```python
from build123d import *

# Parameters (mm, degrees)
F0_W     = 50.8
F0_H     = 25.4
F0_W_2   = 44.45
F0_H_2   = 19.05
F1_DEPTH = 447.675
F2_R     = 3.2385
F2_R_2   = 2.579688
F2_R_3   = 3.175
F3_DEPTH = 25.4
F4_R     = 2.5781
F5_DEPTH = 50.801
F6_DEPTH = 76.2
F7_DEPTH = 25.4


with BuildPart() as f1:
    # F0 (on Front) → F1 (new body)
    with BuildSketch(Plane.XZ):
        with Locations((-27.201447, 17.172885)):
            Rectangle(F0_W, F0_H)
        with Locations((-27.201447, 17.172885)):
            Rectangle(F0_W_2, F0_H_2, mode=Mode.SUBTRACT)
    extrude(amount=F1_DEPTH)

    # F2 (on face) → F3 (cut)
    with BuildSketch(Plane.XY.offset(29.872885)):
        with Locations((-27.201447, -304.8)):
            Circle(F2_R)
        with Locations((-27.201447, -266.7)):
            Circle(F2_R)
        with Locations((-27.201447, -101.6)):
            Circle(F2_R)
        with Locations((-27.201447, -38.1)):
            Circle(F2_R)
        with Locations((-46.251447, -127)):
            Circle(F2_R_2)
        with Locations((-39.901447, -127)):
            Circle(F2_R_2)
        with Locations((-14.501447, -127)):
            Circle(F2_R_2)
        with Locations((-8.151447, -127)):
            Circle(F2_R_2)
        with Locations((-46.251447, -69.85)):
            Circle(F2_R_2)
        with Locations((-39.901447, -69.85)):
            Circle(F2_R_2)
        with Locations((-14.501447, -69.85)):
            Circle(F2_R_2)
        with Locations((-8.151447, -69.85)):
            Circle(F2_R_2)
        with Locations((-43.076447, -238.125)):
            Circle(F2_R_3)
        with Locations((-27.201447, -238.125)):
            Circle(F2_R_3)
        with Locations((-11.326447, -238.125)):
            Circle(F2_R_3)
        with Locations((-12.088447, -388.366)):
            Circle(F2_R_3)
    extrude(amount=-F3_DEPTH, mode=Mode.SUBTRACT)

    # F4 (on face) → F5 (cut, through all)
    with BuildSketch(Plane(origin=(-52.601447, 0, 0), x_dir=(0, -1, 0), z_dir=(-1, 0, 0))):
        with Locations((38.1, 17.172885)):
            Circle(F4_R)
        with Locations((12.7, 17.172885)):
            Circle(F4_R)
        with BuildLine():
            ThreePointArc((60.325, 9.248085), (60.793688, 8.116572), (61.9252, 7.647885))
            Line((61.9252, 7.647885), (77.7748, 7.647885))
            ThreePointArc((77.7748, 7.647885), (78.906312, 8.116572), (79.375, 9.248085))
            Line((79.375, 9.248085), (79.375, 25.097685))
            ThreePointArc((79.375, 25.097685), (78.906312, 26.229197), (77.7748, 26.697885))
            Line((77.7748, 26.697885), (61.9252, 26.697885))
            ThreePointArc((61.9252, 26.697885), (60.793688, 26.229197), (60.325, 25.097685))
            Line((60.325, 25.097685), (60.325, 9.248085))
        make_face()
        with BuildLine():
            ThreePointArc((117.475, 9.248085), (117.943688, 8.116572), (119.0752, 7.647885))
            Line((119.0752, 7.647885), (134.9248, 7.647885))
            ThreePointArc((134.9248, 7.647885), (136.056312, 8.116572), (136.525, 9.248085))
            Line((136.525, 9.248085), (136.525, 25.097685))
            ThreePointArc((136.525, 25.097685), (136.056312, 26.229197), (134.9248, 26.697885))
            Line((134.9248, 26.697885), (119.0752, 26.697885))
            ThreePointArc((119.0752, 26.697885), (117.943688, 26.229197), (117.475, 25.097685))
            Line((117.475, 25.097685), (117.475, 9.248085))
        make_face()
    extrude(amount=-F5_DEPTH, mode=Mode.SUBTRACT)

    # F4 (on face) → F6 (cut)
    with BuildSketch(Plane(origin=(-52.601447, 0, 0), x_dir=(0, -1, 0), z_dir=(-1, 0, 0))):
        with Locations((12.7, 17.172885)):
            Circle(F4_R)
        with Locations((38.1, 17.172885)):
            Circle(F4_R)
        with BuildLine():
            ThreePointArc((60.325, 9.248085), (60.793688, 8.116572), (61.9252, 7.647885))
            Line((61.9252, 7.647885), (77.7748, 7.647885))
            ThreePointArc((77.7748, 7.647885), (78.906312, 8.116572), (79.375, 9.248085))
            Line((79.375, 9.248085), (79.375, 25.097685))
            ThreePointArc((79.375, 25.097685), (78.906312, 26.229197), (77.7748, 26.697885))
            Line((77.7748, 26.697885), (61.9252, 26.697885))
            ThreePointArc((61.9252, 26.697885), (60.793688, 26.229197), (60.325, 25.097685))
            Line((60.325, 25.097685), (60.325, 9.248085))
        make_face()
        with BuildLine():
            ThreePointArc((117.475, 9.248085), (117.943688, 8.116572), (119.0752, 7.647885))
            Line((119.0752, 7.647885), (134.9248, 7.647885))
            ThreePointArc((134.9248, 7.647885), (136.056312, 8.116572), (136.525, 9.248085))
            Line((136.525, 9.248085), (136.525, 25.097685))
            ThreePointArc((136.525, 25.097685), (136.056312, 26.229197), (134.9248, 26.697885))
            Line((134.9248, 26.697885), (119.0752, 26.697885))
            ThreePointArc((119.0752, 26.697885), (117.943688, 26.229197), (117.475, 25.097685))
            Line((117.475, 25.097685), (117.475, 9.248085))
        make_face()
        with BuildLine():
            ThreePointArc((374.65, 23.522885), (376.509872, 19.032757), (381, 17.172885))
            Line((381, 17.172885), (447.675, 17.172885))
            Line((447.675, 17.172885), (447.675, 29.872885))
            Line((447.675, 29.872885), (374.65, 29.872885))
            Line((374.65, 29.872885), (374.65, 23.522885))
        make_face()
    extrude(amount=-F6_DEPTH, mode=Mode.SUBTRACT)

    # F2 (on face) → F7 (cut)
    with BuildSketch(Plane.XY.offset(29.872885)):
        with Locations((-27.963447, -439.801)):
            Circle(F2_R_3)
        with Locations((-43.406647, -432.5366)):
            Circle(F2_R_3)
        with BuildLine():
            Line((-1.801447, -407.543), (-4.976447, -407.543))
            ThreePointArc((-4.976447, -407.543), (-8.151447, -410.718), (-4.976447, -413.893))
            Line((-4.976447, -413.893), (-1.801447, -413.893))
            Line((-1.801447, -413.893), (-1.801447, -407.543))
        make_face()
        with BuildLine():
            Line((-4.976447, -401.701), (-1.801447, -401.701))
            Line((-1.801447, -401.701), (-1.801447, -395.351))
            Line((-1.801447, -395.351), (-4.976447, -395.351))
            ThreePointArc((-4.976447, -395.351), (-8.151447, -398.526), (-4.976447, -401.701))
        make_face()
    extrude(amount=-F7_DEPTH, mode=Mode.SUBTRACT)


solid = f1.part
```
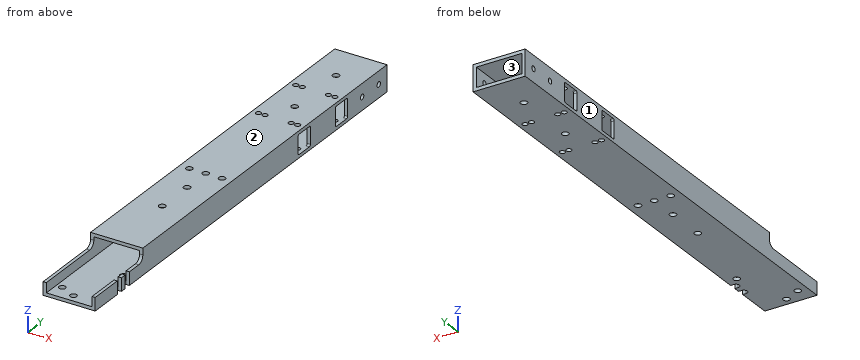
Source: CAD feature listing. Evaluate the final solid. Frame: model axes, mm. Face numbers are marked on the shaded views. Round coordinates to 2 decimals unless told otherwise and drop trailing zeros. Loops run counter-clockwise (first coordinate to the right, second up) from the corner with the lowest first, then second, coordinate; pieces in that order, holes last.
(1) Contact query for flat-ended pins moving along their axis: pin 1 Ø6 at (y, z) = (-38.1, 17.17) entering from -X; pin 2 Ø1.6 at (x, y) = (-3.5, -389.5) entering from +Z. Output: stop coordinate, or through.
From the geometry:
pin 1: stops at x = -52.6
pin 2: stops at z = 17.17
(2) Section query A-A (y = -159). Output: boundary loops of the cut face in (x, z), and give its area (3 significant figures).
From the geometry:
outline: (-52.6, 4.47) - (-1.8, 4.47) - (-1.8, 29.87) - (-52.6, 29.87) - close; hole (-49.43, 7.65) - (-4.98, 7.65) - (-4.98, 26.7) - (-49.43, 26.7) - close
area: 444 mm2
(3) Pull-direction query (Z, two-part tool) for the marked faces 1, 2 and 3; classes: +Z half, -Z half, draft (parallel to the pull), parting line (faces both ways), or undercut.
From the geometry:
face 1: draft
face 2: +Z half
face 3: undercut
(4) Material intervals for probe 1 along Y at (x, z) = (-4, 6.5) (3 decimals); probe 2 along Y at (x, z) = (-4, 14) (3 decimals); probe 3 along Z at (x, y) = (-49, -331.5), sorted ascending.
From the geometry:
probe 1: y = -447.675 to -413.893, -407.543 to -401.701, -395.351 to 0
probe 2: y = -447.675 to -413.893, -407.543 to -401.701, -395.351 to -136.525, -117.475 to -79.375, -60.325 to 0
probe 3: z = 4.47 to 7.65, 26.7 to 29.87
